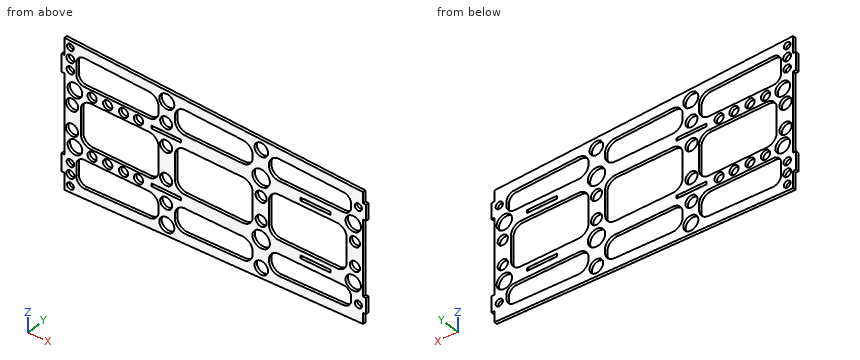
```python
from build123d import *

# Parameters (mm, degrees)
BOSS_EXTRUDE1_DEPTH = 3
SKETCH2_W           = 78
SKETCH2_H           = 45
CUT_EXTRUDE1_DEPTH  = 10
FILLET1_R           = 10
CUT_EXTRUDE2_DEPTH  = 10
SKETCH4_W           = 16.5
SKETCH4_H           = 134.835477832
SKETCH4_H_2         = 126.10677569
BOSS_EXTRUDE2_DEPTH = 3
FILLET2_R           = 10
FILLET3_R           = 10
SKETCH5_W           = 3
SKETCH5_H           = 16
SKETCH5_H_2         = 18
BOSS_EXTRUDE3_DEPTH = 3
SKETCH6_W           = 30
SKETCH6_H           = 3
CUT_EXTRUDE3_DEPTH  = 10
SKETCH7_R           = 7.375435698
SKETCH7_R_2         = 6.026342639
SKETCH7_R_3         = 7.536169895
SKETCH7_R_4         = 8.748796797
SKETCH7_R_5         = 6.84792013
SKETCH7_R_6         = 3.415074188
SKETCH7_R_7         = 4.035175634
SKETCH7_R_8         = 3.768084948
SKETCH7_R_9         = 6.152551264
SKETCH7_R_10        = 4.647289197
SKETCH7_R_11        = 6.093281567
SKETCH7_R_12        = 5.579409228
SKETCH7_R_13        = 7.734472057
SKETCH7_R_14        = 5.13672287
SKETCH7_R_15        = 3.6120817
CUT_EXTRUDE4_DEPTH  = 10


with BuildPart() as part:
    # Sketch1 → Boss-Extrude1 (new body)
    with BuildSketch(Plane(origin=(0, 0, 0), x_dir=(1, 0, 0), z_dir=(0, 1, 0))):
        Polygon((0, 0), (0, 75.000000004), (300, 65), (300, 0), align=None)
    boss_extrude1 = extrude(amount=BOSS_EXTRUDE1_DEPTH)

    # Mirror1: Boss-Extrude1 across Front Plane
    add(boss_extrude1.mirror(Plane.XY))

    # Sketch2 → Cut-Extrude1 (cut)
    with BuildSketch(Plane(origin=(0, 3, 0), x_dir=(1, 0, 0), z_dir=(0, 1, 0))):
        with Locations((55.5, 0)):
            Rectangle(SKETCH2_W, SKETCH2_H)
        with Locations((150, 0)):
            Rectangle(SKETCH2_W, SKETCH2_H)
        with Locations((244.5, 0)):
            Rectangle(SKETCH2_W, SKETCH2_H)
    extrude(amount=-CUT_EXTRUDE1_DEPTH, mode=Mode.SUBTRACT)

    # Fillet1
    fillet1_edges = [part.edges().sort_by_distance(p)[0] for p in [
        (16.5, 1.5, 22.5),
        (16.5, 1.5, -22.5),
        (94.5, 1.5, -22.5),
        (94.5, 1.5, 22.5),
        (111, 1.5, 22.5),
        (111, 1.5, -22.5),
        (189, 1.5, -22.5),
        (189, 1.5, 22.5),
        (205.5, 1.5, 22.5),
        (205.5, 1.5, -22.5),
        (283.5, 1.5, -22.5),
        (283.5, 1.5, 22.5),
    ]]
    fillet(fillet1_edges, radius=FILLET1_R)

    # Sketch3 → Cut-Extrude2 (cut)
    with BuildSketch(Plane(origin=(0, 3, 0), x_dir=(1, 0, 0), z_dir=(0, 1, 0))):
        with BuildLine():
            Line((12, 56.323336113), (12, 44))
            ThreePointArc((12, 44), (14.343145751, 38.343145751), (20, 36))
            Line((20, 36), (280, 36))
            ThreePointArc((280, 36), (285.656854249, 38.343145751), (288, 44))
            Line((288, 44), (288, 47.656669443))
            ThreePointArc((288, 47.656669443), (285.750310824, 53.218496969), (280.266518642, 55.652228699))
            Line((280.266518642, 55.652228699), (20.266518642, 64.318895369))
            ThreePointArc((20.266518642, 64.318895369), (14.438172474, 62.073646937), (12, 56.323336113))
        make_face()
    cut_extrude2 = extrude(amount=-CUT_EXTRUDE2_DEPTH, mode=Mode.SUBTRACT)

    # Mirror2: Cut-Extrude2 across plane
    add(cut_extrude2.mirror(Plane.XY), mode=Mode.SUBTRACT)

    # Sketch4 → Boss-Extrude2 (add)
    with BuildSketch(Plane(origin=(0, 3, 0), x_dir=(1, 0, 0), z_dir=(0, 1, 0))):
        with Locations((102.75, 0)):
            Rectangle(SKETCH4_W, SKETCH4_H)
        with Locations((197.25, 0)):
            Rectangle(SKETCH4_W, SKETCH4_H_2)
    extrude(amount=-BOSS_EXTRUDE2_DEPTH)

    # Fillet2
    fillet2_edges = [part.edges().sort_by_distance(p)[0] for p in [
        (111, 1.5, -36),
        (111, 1.5, -61.294445989),
        (94.5, 1.5, -36),
        (94.5, 1.5, -61.844445989),
        (189, 1.5, -36),
        (205.5, 1.5, -36),
        (205.5, 1.5, -58.144445988),
        (189, 1.5, -58.694445988),
    ]]
    fillet(fillet2_edges, radius=FILLET2_R)

    # Fillet3
    fillet3_edges = [part.edges().sort_by_distance(p)[0] for p in [
        (94.5, 1.5, 36),
        (111, 1.5, 36),
        (111, 1.5, 61.294445989),
        (94.5, 1.5, 61.844445989),
        (189, 1.5, 58.694445988),
        (189, 1.5, 36),
        (205.5, 1.5, 58.144445988),
        (205.5, 1.5, 36),
    ]]
    fillet(fillet3_edges, radius=FILLET3_R)

    # Sketch5 → Boss-Extrude3 (add)
    with BuildSketch(Plane(origin=(0, 3, 0), x_dir=(1, 0, 0), z_dir=(0, 1, 0))):
        with Locations((301.5, 46)):
            Rectangle(SKETCH5_W, SKETCH5_H)
        with Locations((-1.5, 49)):
            Rectangle(SKETCH5_W, SKETCH5_H_2)
        with Locations((301.5, -46)):
            Rectangle(SKETCH5_W, SKETCH5_H)
        with Locations((-1.5, -49)):
            Rectangle(SKETCH5_W, SKETCH5_H_2)
    extrude(amount=-BOSS_EXTRUDE3_DEPTH)

    # Sketch6 → Cut-Extrude3 (cut)
    with BuildSketch(Plane(origin=(0, 3, 0), x_dir=(1, 0, 0), z_dir=(0, 1, 0))):
        with Locations((102.2, 28.5)):
            Rectangle(SKETCH6_W, SKETCH6_H)
        with Locations((252.2, 28.5)):
            Rectangle(SKETCH6_W, SKETCH6_H)
        with Locations((252.2, -28.5)):
            Rectangle(SKETCH6_W, SKETCH6_H)
        with Locations((102.2, -28.5)):
            Rectangle(SKETCH6_W, SKETCH6_H)
    extrude(amount=-CUT_EXTRUDE3_DEPTH, mode=Mode.SUBTRACT)

    # Sketch7 → Cut-Extrude4 (cut)
    with BuildSketch(Plane(origin=(0, 3, 0), x_dir=(1, 0, 0), z_dir=(0, 1, 0))):
        with Locations((10.460573095, 28.013938864)):
            Circle(SKETCH7_R)
        with Locations((102.139763505, 39.635244691)):
            Circle(SKETCH7_R_2)
        with Locations((102.785391607, 60.779565014)):
            Circle(SKETCH7_R_3)
        with Locations((197.531315499, 30.273637219)):
            Circle(SKETCH7_R_4)
        with Locations((197.692722525, 58.197052608)):
            Circle(SKETCH7_R_5)
        with Locations((5.941176384, 68.31573491)):
            Circle(SKETCH7_R_6)
        with Locations((5.941176384, 57.067203431)):
            Circle(SKETCH7_R_7)
        with Locations((5.941176384, 45.768711655)):
            Circle(SKETCH7_R_8)
        with Locations((7.555246638, 12.357457403)):
            Circle(SKETCH7_R_9)
        with Locations((27.731124809, 29.143788042)):
            Circle(SKETCH7_R_10)
        with Locations((43.38760627, 29.143788042)):
            Circle(SKETCH7_R_10)
        with Locations((59.366901782, 29.143788042)):
            Circle(SKETCH7_R_10)
        with Locations((74.377755141, 29.143788042)):
            Circle(SKETCH7_R_10)
        with Locations((102.139763505, 16.325855723)):
            Circle(SKETCH7_R_11)
        with Locations((197.531315499, 11.888841158)):
            Circle(SKETCH7_R_12)
        with Locations((290.098134793, 29.143788042)):
            Circle(SKETCH7_R_13)
        with Locations((291.718609677, 12.12033757)):
            Circle(SKETCH7_R_14)
        with Locations((295.234857663, 47.963698705)):
            Circle(SKETCH7_R_15)
        with Locations((295.234857663, -47.963698705)):
            Circle(SKETCH7_R_15)
        with Locations((291.718609677, -12.12033757)):
            Circle(SKETCH7_R_14)
        with Locations((290.098134793, -29.143788042)):
            Circle(SKETCH7_R_13)
        with Locations((197.531315499, -11.888841158)):
            Circle(SKETCH7_R_12)
        with Locations((102.139763505, -16.325855723)):
            Circle(SKETCH7_R_11)
        with Locations((74.377755141, -29.143788042)):
            Circle(SKETCH7_R_10)
        with Locations((59.366901782, -29.143788042)):
            Circle(SKETCH7_R_10)
        with Locations((43.38760627, -29.143788042)):
            Circle(SKETCH7_R_10)
        with Locations((27.731124809, -29.143788042)):
            Circle(SKETCH7_R_10)
        with Locations((7.555246638, -12.357457403)):
            Circle(SKETCH7_R_9)
        with Locations((5.941176384, -45.768711655)):
            Circle(SKETCH7_R_8)
        with Locations((5.941176384, -57.067203431)):
            Circle(SKETCH7_R_7)
        with Locations((5.941176384, -68.31573491)):
            Circle(SKETCH7_R_6)
        with Locations((197.692722525, -58.197052608)):
            Circle(SKETCH7_R_5)
        with Locations((197.531315499, -30.273637219)):
            Circle(SKETCH7_R_4)
        with Locations((102.785391607, -60.779565014)):
            Circle(SKETCH7_R_3)
        with Locations((102.139763505, -39.635244691)):
            Circle(SKETCH7_R_2)
        with Locations((10.460573095, -28.013938864)):
            Circle(SKETCH7_R)
    extrude(amount=-CUT_EXTRUDE4_DEPTH, mode=Mode.SUBTRACT)


solid = part.part
```
Check sheet for the modelled part. Datum: model origin and axes. Units: mm. Coordinates: 2 decimals unless noted, no trailing zeros. Write each loop counter-clockwise with the first axis right and the second up, starting at its lowest first coordinate (ties: lowest second). Pieces come first, ordered by that corner, then holes. Notation, with made-up numbers: (-4.75, 52.5) - (39.25, 52.5) arc R21 ccw to (39.25, 82.5) - close; hole circle Ø3 at (63.25, 89). An arc over 180 degrees is marked (long way). One line per question, with ' | ' between items.
Item 1: Gauge pin test, flat ends, axial feed: P1, Ø1.5, axis at y = 1, z = -4, coming from the -X side; P2, Ø1.5, axis at x = 43.5, y = 2, coming from the +Z side (3 decimals); P3, Ø9.5, axis at x = 295.23, z = 47.96, coming from the -Y side. Record the tip position at first contact, or that the pin passes through.
Determined:
P1: stops at x = 0 | P2: stops at z = 73.575 | P3: stops at y = 0
Item 2: Sectioned sample at B-B on x = 139.5. Record the boundary of the cut face in (y, z).
Determined:
outline: (0, -70.35) - (3, -70.35) - (3, -60.34) - (0, -60.34) - close; (0, -36) - (3, -36) - (3, -22.5) - (0, -22.5) - close; (0, 22.5) - (3, 22.5) - (3, 36) - (0, 36) - close; (0, 60.34) - (3, 60.34) - (3, 70.35) - (0, 70.35) - close
Item 3: Sectioned sample at D-D on y = 1.75. Give the number of separate pieces and of enclosed holes in the cut face, plus the area to 3 significant figures.
Determined:
separate pieces: 1 | enclosed holes: 49 | area: 16,600 mm2
Item 4: Sectioned sample at C-C on x = 58.5. Record the boundary of the cut face in (y, z).
Determined:
outline: (0, -73.05) - (3, -73.05) - (3, -63.04) - (0, -63.04) - close; (0, -36) - (3, -36) - (3, -33.71) - (0, -33.71) - close; (0, -24.58) - (3, -24.58) - (3, -22.5) - (0, -22.5) - close; (0, 22.5) - (3, 22.5) - (3, 24.58) - (0, 24.58) - close; (0, 33.71) - (3, 33.71) - (3, 36) - (0, 36) - close; (0, 63.04) - (3, 63.04) - (3, 73.05) - (0, 73.05) - close
Item 5: Sectioned sample at A-A on x = 246. Record the boundary of the cut face in (y, z).
Determined:
outline: (0, -66.8) - (3, -66.8) - (3, -56.79) - (0, -56.79) - close; (0, -36) - (3, -36) - (3, -30) - (0, -30) - close; (0, -27) - (3, -27) - (3, -22.5) - (0, -22.5) - close; (0, 22.5) - (3, 22.5) - (3, 27) - (0, 27) - close; (0, 30) - (3, 30) - (3, 36) - (0, 36) - close; (0, 56.79) - (3, 56.79) - (3, 66.8) - (0, 66.8) - close
Item 6: Thickness scan on line 1 (X direction, y = 2.65, z = -5.5); line 2 (Z direction, x = 189.5, y = 2.55); line 3 (Z direction, x = 46.5, y = 1.75). Record the ranges inside material, lowest first. Write a range as [from, to].
Determined:
line 1: x = [0, 16.5], [94.5, 111], [189, 205.5], [283.5, 300] | line 2: z = [-68.68, -33.74], [-26.8, 26.8], [33.74, 68.68] | line 3: z = [-73.45, -63.44], [-36, -32.59], [-25.69, -22.5], [22.5, 25.69], [32.59, 36], [63.44, 73.45]
